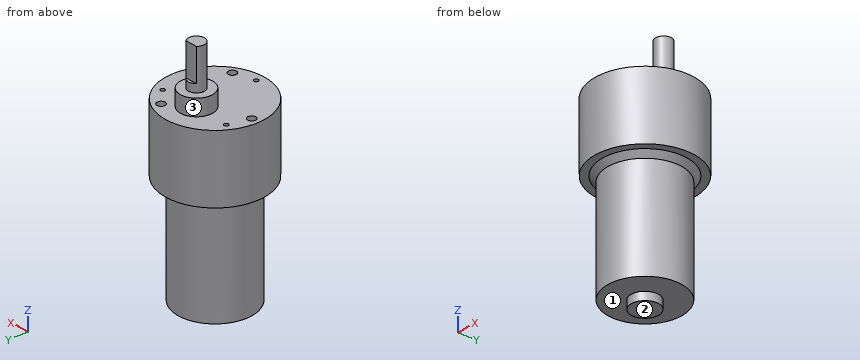
```python
from build123d import *

# Parameters (mm, degrees)
SKETCH_2_R          = 13.75
EXTRUDE_1_DEPTH     = 40
SKETCH_3_R          = 18.5
EXTRUDE_2_DEPTH     = 25
CHAMFER_1_SIZE      = 2
SKETCH_4_R          = 6
EXTRUDE_3_DEPTH     = 6
SKETCH_5_R          = 3
EXTRUDE_4_DEPTH     = 15
CUT_EXTRUDE_1_DEPTH = 12
SKETCH_7_R          = 1.5
CUT_EXTRUDE_2_DEPTH = 6
SKETCH_8_R          = 1.5
CUT_EXTRUDE_3_DEPTH = 6
SKETCH_10_R         = 1.5
CUT_EXTRUDE_4_DEPTH = 6
SKETCH_11_R         = 5.1
EXTRUDE_5_DEPTH     = 3
M2X0_4_1_D          = 1.6
M2X0_4_1_DEPTH      = 6
M2X0_4_1_TIP        = 0.480688495


with BuildPart() as part:
    # ｽｹｯﾁ2 → ﾎﾞｽ - 押し出し1 (new body)
    with BuildSketch(Plane.XY):
        Circle(SKETCH_2_R)
    extrude(amount=EXTRUDE_1_DEPTH)

    # ｽｹｯﾁ3 → ﾎﾞｽ - 押し出し2 (add)
    with BuildSketch(Plane.XY.offset(40)):
        Circle(SKETCH_3_R)
    extrude(amount=EXTRUDE_2_DEPTH)

    # 面取り1
    chamfer_1_edges = [part.edges().sort_by_distance(p)[0] for p in [
        (-13.75, 0, 40),
    ]]
    chamfer(chamfer_1_edges, length=CHAMFER_1_SIZE)

    # ｽｹｯﾁ4 → ﾎﾞｽ - 押し出し3 (add)
    with BuildSketch(Plane.XY.offset(65)):
        with Locations((0, 7)):
            Circle(SKETCH_4_R)
    extrude(amount=EXTRUDE_3_DEPTH)

    # ｽｹｯﾁ5 → ﾎﾞｽ - 押し出し4 (add)
    with BuildSketch(Plane.XY.offset(71)):
        with Locations((0, 7)):
            Circle(SKETCH_5_R)
    extrude(amount=EXTRUDE_4_DEPTH)

    # ｽｹｯﾁ6 → ｶｯﾄ - 押し出し1 (cut)
    with BuildSketch(Plane.XY.offset(86)):
        with BuildLine():
            Line((-2.222509648, 9.015056045), (2.222509648, 9.015056045))
            ThreePointArc((2.222509648, 9.015056045), (0, 10), (-2.222509648, 9.015056045))
        make_face()
    extrude(amount=-CUT_EXTRUDE_1_DEPTH, mode=Mode.SUBTRACT)

    # ｽｹｯﾁ7 → ｶｯﾄ - 押し出し2 (cut)
    with BuildSketch(Plane.XY.offset(65)):
        with Locations((-15.5, 0)):
            Circle(SKETCH_7_R)
    extrude(amount=-CUT_EXTRUDE_2_DEPTH, mode=Mode.SUBTRACT)

    # ｽｹｯﾁ8 → ｶｯﾄ - 押し出し3 (cut)
    with BuildSketch(Plane.XY.offset(65)):
        with Locations((7.75, -13.423393759)):
            Circle(SKETCH_8_R)
    extrude(amount=-CUT_EXTRUDE_3_DEPTH, mode=Mode.SUBTRACT)

    # ｽｹｯﾁ10 → ｶｯﾄ - 押し出し4 (cut)
    with BuildSketch(Plane.XY.offset(65)):
        with Locations((7.75, 13.423393759)):
            Circle(SKETCH_10_R)
    extrude(amount=-CUT_EXTRUDE_4_DEPTH, mode=Mode.SUBTRACT)

    # ｽｹｯﾁ11 → ﾎﾞｽ - 押し出し5 (add)
    with BuildSketch(Plane(origin=(0, 0, 0), x_dir=(-1, 0, 0), z_dir=(0, 0, -1))):
        Circle(SKETCH_11_R)
    extrude(amount=EXTRUDE_5_DEPTH)

    # M2x0.4 ねじ穴1
    with Locations(Plane.XY.offset(65)):
        with Locations((-13.423393759, 7.75), (0, -15.5), (13.423393759, 7.75)):
            Hole(M2X0_4_1_D / 2, depth=M2X0_4_1_DEPTH)
            with Locations((0, 0, -(M2X0_4_1_DEPTH + M2X0_4_1_TIP / 2))):  # 118° drill point
                Cone(0, M2X0_4_1_D / 2, M2X0_4_1_TIP, mode=Mode.SUBTRACT)


solid = part.part
```
Geometry check sheet. Reference: the model listing, model coordinates, mm. Face numbers are marked on the shaded views. A direction names the side the tool comes from. Give positions to 0.01 mm unless a question says otherwise; leave off trailing zeros. Write each loop counter-clockwise with the first axis right and the second up, starting at its lowest first coordinate (ties: lowest second). Pieces come first, ordered by that corner, then holes. Notation, with made-up numbers: (59.25, 50.25) - (106.25, 50.25) arc R8 cw to (106.25, 59.25) - close; hole circle Ø2 at (67.5, 57.5). An arc over 180 degrees is marked (long way). Use a Markdown table: item, result.
Q1. Section check A-A, the plane y = 0. Enter the section's corners in (x, z).
Computed:
| item | result |
|---|---|
| outline | (-18.5, 40) - (-15.75, 40) - (-13.75, 38) - (-13.75, 0) - (-5.1, 0) - (-5.1, -3) - (5.1, -3) - (5.1, 0) - (13.75, 0) - (13.75, 38) - (15.75, 40) - (18.5, 40) - (18.5, 65) - (-14, 65) - (-14, 59) - (-17, 59) - (-17, 65) - (-18.5, 65) - close |
Q2. Thickness scan on L1, parallel to Y at x = 0, z = 61.6; L2, parallel to X at y = 7.75, z = 62.5; L3, parallel to Z at x = 6, y = -2. Record the ranges inside material, lowest first. Write a range as [from, to].
Computed:
| item | result |
|---|---|
| L1 | y = [-18.5, -16.3], [-14.7, 18.5] |
| L2 | x = [-16.8, -14.22], [-12.62, 12.62], [14.22, 16.8] |
| L3 | z = [0, 65] |
Q3. Set-up check for the marked faces 1, 2 and 3: record each of +Z, -Z, +X, -X, +Y, -Y from which the full face is reachable in a straight line by a thin tool's end or side.
Computed:
| item | result |
|---|---|
| face 1 | -Z |
| face 2 | -Z, +X, -X, +Y, -Y |
| face 3 | +Z |
Q4. Section check B-B, the plane z = 53. Enter the section's corners in (x, y).
Computed:
| item | result |
|---|---|
| outline | circle Ø37 at (0, 0) |
Q5. Go/stop test with flat-tipped pins: P1, Ø3, axis at x = -14.5, z = 44, coming from the -Y side; P2, Ø8, axis at x = 10.5, z = 42.5, coming from the -Y side; P3, Ø1.8, axis at x = 0, y = -15.5, coming from the +Z side; P4, Ø18.5, axis at x = 1, y = 8.5, coming from the -Z side. Record where each tip stops, or that it passes through.
Computed:
| item | result |
|---|---|
| P1 | stops at y = -13.16 |
| P2 | stops at y = -17.32 |
| P3 | stops at z = 65 |
| P4 | stops at z = -3 |
